from build123d import *

# Parameters (mm, degrees)
SKETCH1_R           = 2.55
BOSS_EXTRUDE1_DEPTH = 5
BOSS_EXTRUDE2_DEPTH = 20
BOSS_EXTRUDE3_DEPTH = 15
CUT_EXTRUDE1_DEPTH  = 39.418745425


with BuildPart() as part:
    # Sketch1 → Boss-Extrude1 (new body)
    # profile 1 of 2: a face of its own
    with BuildSketch(Plane(origin=(0, 0, 0), x_dir=(1, 0, 0), z_dir=(0, 1, 0))):
        with BuildLine():
            Line((6.075398109, 20), (0, 20))
            Line((0, 20), (0, 0))
            Line((0, 0), (20, 0))
            Line((20, 0), (20, 20))
            Line((20, 20), (13.924601891, 20))
            ThreePointArc((13.924601891, 20), (10, 16.95), (6.075398109, 20))
        make_face()
        with Locations(Location((10, 10, 0), (0, 0, 270))):
            Circle(SKETCH1_R, mode=Mode.SUBTRACT)
    # profile 2 of 2: a face of its own
    with BuildSketch(Plane(origin=(0, 0, 0), x_dir=(1, 0, 0), z_dir=(0, 1, 0))):
        with BuildLine():
            Line((0, 26), (0, 20))
            Line((0, 20), (6.075398109, 20))
            ThreePointArc((6.075398109, 20), (9.496084162, 25.018528192), (14.05, 21))
            ThreePointArc((14.05, 21), (14.018528192, 20.496084162), (13.924601891, 20))
            Line((13.924601891, 20), (20, 20))
            Line((20, 20), (20, 26))
            Line((20, 26), (0, 26))
        make_face()
    extrude(amount=BOSS_EXTRUDE1_DEPTH)

    # Sketch1<3> → Boss-Extrude2 (add)
    with BuildSketch(Plane(origin=(0, 0, 0), x_dir=(1, 0, 0), z_dir=(0, 1, 0))):
        with BuildLine():
            Line((0, 26), (0, 20))
            Line((0, 20), (6.075398109, 20))
            ThreePointArc((6.075398109, 20), (9.496084162, 25.018528192), (14.05, 21))
            ThreePointArc((14.05, 21), (14.018528192, 20.496084162), (13.924601891, 20))
            Line((13.924601891, 20), (20, 20))
            Line((20, 20), (20, 26))
            Line((20, 26), (0, 26))
        make_face()
    extrude(amount=BOSS_EXTRUDE2_DEPTH)

    # Sketch3 → Boss-Extrude3 (add)
    with BuildSketch(Plane(origin=(0, 5, 0), x_dir=(1, 0, 0), z_dir=(0, 1, 0))):
        with BuildLine():
            Line((13.924601891, 20), (6.075398109, 20))
            ThreePointArc((6.075398109, 20), (10, 25.05), (13.924601891, 20))
        make_face()
    extrude(amount=BOSS_EXTRUDE3_DEPTH)

    # Sketch2 → Cut-Extrude1 (cut, through all)
    with BuildSketch(Plane(origin=(0, 0, -26), x_dir=(-1, 0, 0), z_dir=(0, 0, -1))):
        with BuildLine():
            ThreePointArc((-12.55, 12.5), (-10, 9.95), (-7.45, 12.5))
            Line((-7.45, 12.5), (-12.55, 12.5))
        make_face()
        with BuildLine():
            Line((-12.55, 12.5), (-7.45, 12.5))
            ThreePointArc((-7.45, 12.5), (-10, 15.05), (-12.55, 12.5))
        make_face()
    extrude(amount=-CUT_EXTRUDE1_DEPTH, mode=Mode.SUBTRACT)


solid = part.part
Could you check a few things on this model? Use its own coordinates, in mm. A direction names the side the tool comes from. Give positions to 0.01 mm unless a question says otherwise; leave off trailing zeros. Order: outer loops, then holes, each group sorted by start corner. A loop starts at its lowest first (then second) coordinate and runs counter-clockwise, first axis right, second up.
1. Will these pins go through, and if not, where does the flat tip stop? P1, Ø1, axis at y = 6.5, z = -14.5, coming from the -X side; P2, Ø5.5, axis at x = 10.5, z = -21.5, coming from the -Y side; P3, Ø4.5, axis at x = 5.5, y = 11.5, coming from the +Z side; P4, Ø6, axis at x = 13, z = -13.5, coming from the +Y side.
2. I need wall thicknesses on L1, parallel to X at y = 2.4, z = -10; L2, parallel to X at y = 3.55, z = -21; L3, parallel to Y at x = 10, z = -22.8. Which ranges of each line are inside material? Lowest first, please.
3. Suppose I cut it at D-D (x = 15). List the corners of the cut face in (y, z) for me.
4. Suppose I cut it at B-B (y = 12.5). List the corners of the cut face in (x, z) for me.
5. For faces 1 (the flat face through (10, 5, -22)), 2 (the flat face through (10, 20, -23)), 3 (the flat face through (12.4, 10.7, -20)), which set-ups out of +Z, -Z, +X, -X, +Y, -Y let a thin tool reach every point of the face, with its end or its side?
6. Suppose I cut it at A-A (z = -10). List the corners of the cut face in (x, y) for me.
7. Suppose I cut it at C-C (y = 2.25). List the corners of the cut face in (x, z) for me.
8. We'd pull the mould along Y, two halves only. Please class faces 4 (the flat face through (12, 5, -8)), 5 (the cylindrical face through (10.55, 10.01, -23.04)), 6 (the flat face through (20, 3, -19)): pulls with the +Y half, pulls with the -Y half, needs draft (parallel to the pull), parting line crosses it, or undercut.
Solved:
1. P1: passes through
1. P2: stops at y = 5
1. P3: stops at z = -20
1. P4: stops at y = 5
2. L1: x = 0 to 7.45, 12.55 to 20
2. L2: x = 0 to 5.95, 14.05 to 20
2. L3: y = 5 to 9.95, 15.05 to 20
3. outline: (0, -26) - (20, -26) - (20, -20) - (5, -20) - (5, 0) - (0, 0) - close
4. outline: (0, -26) - (7.45, -26) - (7.45, -20) - (0, -20) - close; (12.55, -26) - (20, -26) - (20, -20) - (12.55, -20) - close
5. face 1: -Y
5. face 2: +Z, -Z, +X, -X, +Y
5. face 3: +Z, +X, -X, +Y
6. outline: (0, 0) - (7.45, 0) - (7.45, 5) - (0, 5) - close; (12.55, 0) - (20, 0) - (20, 5) - (12.55, 5) - close
7. outline: (0, -26) - (20, -26) - (20, 0) - (0, 0) - close; hole circle Ø8.1 at (10, -21); hole circle Ø5.1 at (10, -10)
8. face 4: pulls with the +Y half
8. face 5: undercut
8. face 6: needs draft
